Model file for the job. Use its own axes, mm. Coordinates: 2 decimals unless noted, no trailing zeros. Loops run counter-clockwise (first coordinate to the right, second up) from the corner with the lowest first, then second, coordinate; pieces in that order, holes last. Notation, with made-up numbers: M 76,-3.5 L 80,-3.5 A27 cw 80,30.5 Z; hole C 48.25,81 d11. An arc over 180 degrees is marked long. One line per question, with ' | ' between items. Start each with the question number.
```python
from build123d import *

# Parameters (mm, degrees)
MODEL_R         = 11
MODEL_R_2       = 2.1
MODEL_R_3       = 2.625
EXTRUDE_1_DEPTH = 4


with BuildPart() as part:
    # Model → 凸台-拉伸1 (new body)
    with BuildSketch(Plane.XY):
        with BuildLine():
            Line((-80, 70), (-116, 70))
            ThreePointArc((-116, 70), (-117.414213562, 69.414213562), (-118, 68))
            Line((-118, 68), (-118, -20))
            ThreePointArc((-118, -20), (-115.071067812, -27.071067812), (-108, -30))
            Line((-108, -30), (31, -30))
            ThreePointArc((31, -30), (32.414213562, -29.414213562), (33, -28))
            Line((33, -28), (33, 28))
            ThreePointArc((33, 28), (32.414213562, 29.414213562), (31, 30))
            Line((31, 30), (-68, 30))
            ThreePointArc((-68, 30), (-75.071067812, 32.928932188), (-78, 40))
            Line((-78, 40), (-78, 68))
            ThreePointArc((-78, 68), (-78.585786438, 69.414213562), (-80, 70))
        make_face()
        with Locations((-98, 50)):
            Circle(MODEL_R, mode=Mode.SUBTRACT)
        with Locations((-110, 62)):
            Circle(MODEL_R_2, mode=Mode.SUBTRACT)
        with Locations((-86, 62)):
            Circle(MODEL_R_2, mode=Mode.SUBTRACT)
        with Locations((-110, 38)):
            Circle(MODEL_R_2, mode=Mode.SUBTRACT)
        with Locations((-86, 38)):
            Circle(MODEL_R_2, mode=Mode.SUBTRACT)
        with Locations((-61.5, 8)):
            Circle(MODEL_R_3, mode=Mode.SUBTRACT)
        with Locations((-41.5, 8)):
            Circle(MODEL_R_3, mode=Mode.SUBTRACT)
        with Locations((-41.5, -22)):
            Circle(MODEL_R_3, mode=Mode.SUBTRACT)
        with Locations((-61.5, -22)):
            Circle(MODEL_R_3, mode=Mode.SUBTRACT)
        with Locations((-108, 8)):
            Circle(MODEL_R_3, mode=Mode.SUBTRACT)
        with Locations((-88, 8)):
            Circle(MODEL_R_3, mode=Mode.SUBTRACT)
        with Locations((-108, -22)):
            Circle(MODEL_R_3, mode=Mode.SUBTRACT)
        with Locations((-88, -22)):
            Circle(MODEL_R_3, mode=Mode.SUBTRACT)
        with BuildLine():
            Line((-20.5, -20.875), (-26.5, -20.875))
            ThreePointArc((-26.5, -20.875), (-29.125, -23.5), (-26.5, -26.125))
            Line((-26.5, -26.125), (-20.5, -26.125))
            ThreePointArc((-20.5, -26.125), (-17.875, -23.5), (-20.5, -20.875))
        make_face(mode=Mode.SUBTRACT)
        with BuildLine():
            Line((20.5, 20.875), (26.5, 20.875))
            ThreePointArc((26.5, 20.875), (29.125, 23.5), (26.5, 26.125))
            Line((26.5, 26.125), (20.5, 26.125))
            ThreePointArc((20.5, 26.125), (17.875, 23.5), (20.5, 20.875))
        make_face(mode=Mode.SUBTRACT)
        with BuildLine():
            Line((-3, -19.05), (3, -19.05))
            ThreePointArc((3, -19.05), (22.05, 0), (3, 19.05))
            Line((3, 19.05), (-3, 19.05))
            ThreePointArc((-3, 19.05), (-22.05, 0), (-3, -19.05))
        make_face(mode=Mode.SUBTRACT)
        with BuildLine():
            Line((-26.5, 20.875), (-20.5, 20.875))
            ThreePointArc((-20.5, 20.875), (-17.875, 23.5), (-20.5, 26.125))
            Line((-20.5, 26.125), (-26.5, 26.125))
            ThreePointArc((-26.5, 26.125), (-29.125, 23.5), (-26.5, 20.875))
        make_face(mode=Mode.SUBTRACT)
        with BuildLine():
            Line((26.5, -20.875), (20.5, -20.875))
            ThreePointArc((20.5, -20.875), (17.875, -23.5), (20.5, -26.125))
            Line((20.5, -26.125), (26.5, -26.125))
            ThreePointArc((26.5, -26.125), (29.125, -23.5), (26.5, -20.875))
        make_face(mode=Mode.SUBTRACT)
    extrude(amount=EXTRUDE_1_DEPTH)


solid = part.part
```
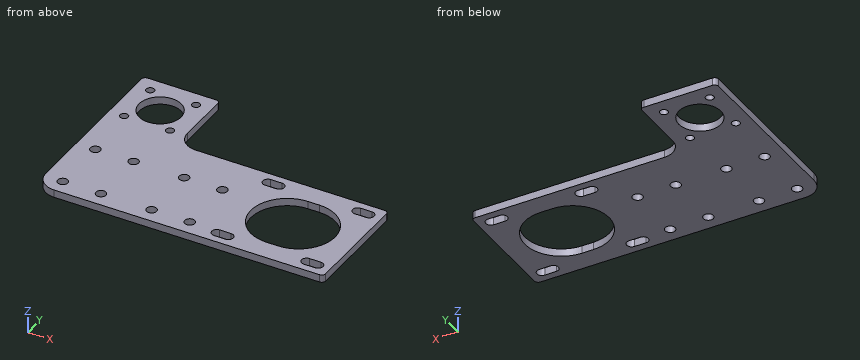
(1) Pin check, flat tip, straight feed: P1, Ø1.2, axis at x = 23, z = 1, coming from the +Y side. Stop position of the tip, or through.
(2) Drill centre lines: line 1 (Y direction, x = -41.5, z = 3.15) (3 decimals); line 2 (Y direction, x = -86, z = 1.35); line 3 (X direction, y = -1, z = 0.3). Where is each one in solid material? Low to high. Write a range as [from, to].
(3) Band-saw the part on A-A on y = 50. Write the cut outline in (x, z).
(4) Band-saw the part on B-B on y = 23.5. Write the cut outline in (x, z) (3 decimals).
(5) Band-saw the part on D-D on z = 0.7. Give the number of separate pieces and of enclosed holes in the cut face, then the cut area to 3 significant figures.
(6) Band-saw the part on C-C on y = 8. Write the cut outline in (x, z) (3 decimals).
Computed values:
1) P1: y = 30
2) line 1: [-30, -24.625], [-19.375, 5.375], [10.625, 30] | line 2: [-30, -23.7], [-20.3, 6.3], [9.7, 35.9], [40.1, 59.9], [64.1, 70] | line 3: [-118, -22.02], [22.02, 33]
3) outline: M -118,0 L -109,0 L -109,4 L -118,4 Z; M -87,0 L -78,0 L -78,4 L -87,4 Z
4) outline: M -118,0 L -29.125,0 L -29.125,4 L -118,4 Z; M -17.875,0 L 17.875,0 L 17.875,4 L -17.875,4 Z; M 29.125,0 L 33,0 L 33,4 L 29.125,4 Z
5) separate pieces: 1 | enclosed holes: 18 | area: 8,470 mm^2
6) outline: M -118,0 L -110.625,0 L -110.625,4 L -118,4 Z; M -105.375,0 L -90.625,0 L -90.625,4 L -105.375,4 Z; M -85.375,0 L -64.125,0 L -64.125,4 L -85.375,4 Z; M -58.875,0 L -44.125,0 L -44.125,4 L -58.875,4 Z; M -38.875,0 L -20.289,0 L -20.289,4 L -38.875,4 Z; M 20.289,0 L 33,0 L 33,4 L 20.289,4 Z
